Read the model definition and answer for the solid it produces. Units are mm, in the model's axes. Round coordinates to 2 decimals unless told otherwise and drop trailing zeros. Order: outer loops, then holes, each group sorted by start corner. A loop starts at its lowest first (then second) coordinate and runs counter-clockwise, first axis right, second up. Notation, with made-up numbers: (14.25, 56.25) - (44.25, 56.25) arc R5 ccw to (44.25, 63.25) - close; hole circle Ø8 at (-35, 81.5). An arc over 180 degrees is marked (long way). One line per question, with ' | ' between items. Start each with the question number.
1) A flat-ended cylindrical pin translates along its axis: pin 1 (3 mm diameter, centred on x = 129.5, y = -14.5, fed in from +Z). Find the tip coordinate at first contact, or state that the pin passes through.
2) The part is cut by section A-A, the plane x = 273. Give the vertices of the cut face in (y, z).
3) Straight lines are drawn through the part: line 1 (Y direction, x = 370, z = 11.25); line 2 (Y direction, x = 310, z = 8.5); line 3 (Z direction, x = 18.5, y = -8.5). For each, find the intervals that lie inside material, in ascending order. Write a range as from..to.
from build123d import *

# Parameters (mm, degrees)
F1_DEPTH = 400
F2_R     = 3
F3_DEPTH = 18
F4_R     = 5
F5_DEPTH = 7


with BuildPart() as f1:
    # F0 (on Right) → F1 (new body)
    with BuildSketch(Plane.YZ):
        with BuildLine():
            Line((-26.041336, 5), (-26.041336, 0))
            Line((-26.041336, 0), (-6.041336, 0))
            Line((-6.041336, 0), (-6.041336, 5))
            ThreePointArc((-6.041336, 5), (-9.041336, 8), (-6.041336, 11))
            Line((-6.041336, 11), (-6.041336, 15))
            ThreePointArc((-6.041336, 15), (-8.162657, 15.87868), (-9.041336, 18))
            Line((-9.041336, 18), (-23.041336, 18))
            ThreePointArc((-23.041336, 18), (-23.920016, 15.87868), (-26.041336, 15))
            Line((-26.041336, 15), (-26.041336, 11))
            ThreePointArc((-26.041336, 11), (-23.041336, 8), (-26.041336, 5))
        make_face()
    extrude(amount=F1_DEPTH)

    # F2 (on face) → F3 (cut)
    with BuildSketch(Plane.XY.offset(18)):
        with Locations((10, -16.041336)):
            Circle(F2_R)
        with Locations((70, -16.041336)):
            Circle(F2_R)
        with Locations((130, -16.041336)):
            Circle(F2_R)
        with Locations((190, -16.041336)):
            Circle(F2_R)
        with Locations((250, -16.041336)):
            Circle(F2_R)
        with Locations((310, -16.041336)):
            Circle(F2_R)
        with Locations((370, -16.041336)):
            Circle(F2_R)
        with Locations((430, -16.041336)):
            Circle(F2_R)
        with Locations((490, -16.041336)):
            Circle(F2_R)
        with Locations((550, -16.041336)):
            Circle(F2_R)
        with Locations((610, -16.041336)):
            Circle(F2_R)
        with Locations((670, -16.041336)):
            Circle(F2_R)
        with Locations((730, -16.041336)):
            Circle(F2_R)
        with Locations((790, -16.041336)):
            Circle(F2_R)
        with Locations((850, -16.041336)):
            Circle(F2_R)
        with Locations((910, -16.041336)):
            Circle(F2_R)
        with Locations((970, -16.041336)):
            Circle(F2_R)
        with Locations((1030, -16.041336)):
            Circle(F2_R)
        with Locations((1090, -16.041336)):
            Circle(F2_R)
        with Locations((1150, -16.041336)):
            Circle(F2_R)
        with Locations((1210, -16.041336)):
            Circle(F2_R)
        with Locations((1270, -16.041336)):
            Circle(F2_R)
        with Locations((1330, -16.041336)):
            Circle(F2_R)
        with Locations((1390, -16.041336)):
            Circle(F2_R)
        with Locations((1450, -16.041336)):
            Circle(F2_R)
        with Locations((1510, -16.041336)):
            Circle(F2_R)
        with Locations((1570, -16.041336)):
            Circle(F2_R)
        with Locations((1630, -16.041336)):
            Circle(F2_R)
        with Locations((1690, -16.041336)):
            Circle(F2_R)
        with Locations((1750, -16.041336)):
            Circle(F2_R)
        with Locations((1810, -16.041336)):
            Circle(F2_R)
        with Locations((1870, -16.041336)):
            Circle(F2_R)
        with Locations((1930, -16.041336)):
            Circle(F2_R)
        with Locations((1990, -16.041336)):
            Circle(F2_R)
    extrude(amount=-F3_DEPTH, mode=Mode.SUBTRACT)

    # F4 (on face) → F5 (cut)
    with BuildSketch(Plane.XY.offset(18)):
        with Locations((10, -16.041336)):
            Circle(F4_R)
        with Locations((70, -16.041336)):
            Circle(F4_R)
        with Locations((130, -16.041336)):
            Circle(F4_R)
        with Locations((190, -16.041336)):
            Circle(F4_R)
        with Locations((250, -16.041336)):
            Circle(F4_R)
        with Locations((310, -16.041336)):
            Circle(F4_R)
        with Locations((370, -16.041336)):
            Circle(F4_R)
    extrude(amount=-F5_DEPTH, mode=Mode.SUBTRACT)


solid = f1.part
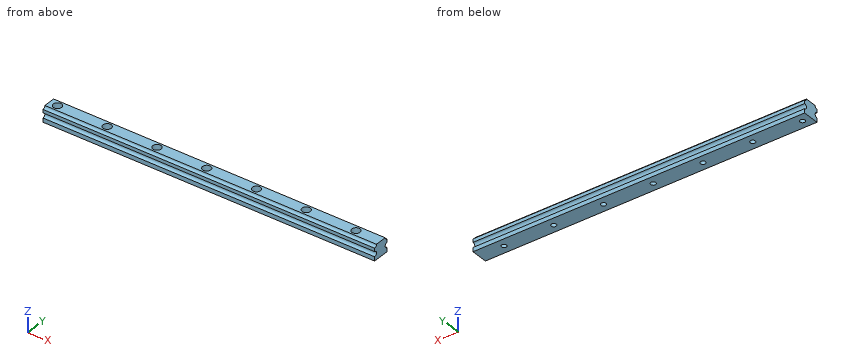
Values:
1) pin 1: stops at z = 11
2) outline: (-26.04, 0) - (-6.04, 0) - (-6.04, 5) arc R3 cw to (-6.04, 11) - (-6.04, 15) arc R3 cw to (-9.04, 18) - (-23.04, 18) arc R3 cw to (-26.04, 15) - (-26.04, 11) arc R3 cw to (-26.04, 5) - close
3) line 1: y = -26.04..-21.04, -11.04..-6.04 | line 2: y = -23.08..-19.04, -13.04..-9 | line 3: z = 0..6.28, 9.72..16.28
